from build123d import *

# Parameters (mm, degrees)
SKETCH_1_W          = 4
SKETCH_1_H          = 15
SKETCH_2_R          = 12
EXTRUDE_1_DEPTH     = 25
SKETCH_3_R          = 11
EXTRUDE_2_DEPTH     = 31
SKETCH_4_R          = 10
EXTRUDE_3_DEPTH     = 25
CUT_EXTRUDE_1_DEPTH = 3
CHAMFER_1_SIZE      = 1
FILLET_1_R          = 1


with BuildPart() as part:
    # Эскиз1 → Повернуть1 (revolve)
    with BuildSketch(Plane.XY, mode=Mode.PRIVATE) as revolve_1_sk:
        with Locations((2, 7.5)):
            Rectangle(SKETCH_1_W, SKETCH_1_H)
    revolve(revolve_1_sk.sketch.rotate(Axis((0, 0, 0), (1, 0, 0)), 270), axis=Axis((0, 0, 0), (1, 0, 0)))

    # Эскиз2 → Бобышка-Вытянуть1 (add)
    with BuildSketch(Plane(origin=(4, 0, 0), x_dir=(0, 0, -1), z_dir=(1, 0, 0))):
        Circle(SKETCH_2_R)
    extrude(amount=EXTRUDE_1_DEPTH)

    # Эскиз3 → Бобышка-Вытянуть2 (add)
    with BuildSketch(Plane(origin=(29, 0, 0), x_dir=(0, 0, -1), z_dir=(1, 0, 0))):
        Circle(SKETCH_3_R)
    extrude(amount=EXTRUDE_2_DEPTH)

    # Эскиз4 → Бобышка-Вытянуть3 (add)
    with BuildSketch(Plane(origin=(60, 0, 0), x_dir=(0, 0, -1), z_dir=(1, 0, 0))):
        Circle(SKETCH_4_R)
    extrude(amount=EXTRUDE_3_DEPTH)

    # Эскиз5 → Вырез-Вытянуть1 (cut)
    with BuildSketch(Plane(origin=(80, 0, 0), x_dir=(0, -1, 0), z_dir=(-1, 0, 0))):
        with BuildLine():
            Line((7.141428429, -7), (-7.141428429, -7))
            ThreePointArc((-7.141428429, -7), (0, -10), (7.141428429, -7))
        make_face()
    extrude(amount=-CUT_EXTRUDE_1_DEPTH, mode=Mode.SUBTRACT)

    # Фаска1
    chamfer_1_edges = [part.edges().sort_by_distance(p)[0] for p in [
        (85, 0, 10),
        (0, 0, 15),
    ]]
    chamfer(chamfer_1_edges, length=CHAMFER_1_SIZE)

    # Скругление1
    fillet_1_edges = [part.edges().sort_by_distance(p)[0] for p in [
        (4, 0, 12),
    ]]
    fillet(fillet_1_edges, radius=FILLET_1_R)


solid = part.part
For this review, take the finished solid that the model builds, in its own axes (mm). A direction names the side the tool comes from. Round coordinates to 2 decimals unless told otherwise and drop trailing zeros. Write each loop counter-clockwise with the first axis right and the second up, starting at its lowest first coordinate (ties: lowest second). Pieces come first, ordered by that corner, then holes. Notation, with made-up numbers: M 41,-31 L 69,-31 A14 cw 69,-5 Z; hole C 70.5,29.5 d3. An arc over 180 degrees is marked long. Write item = value, one per line. Start each with the question number.
(1) The part is to be moulded in two halves that separate along X. For faces 1 (the face through (80, 0, -8)), 2 (the face through (60, -10, -2)), 3 (the face through (44.28, -10.74, 2.38)), say which applies: +X half, -X half, draft (parallel to the pull), parting line (faces both ways), or undercut.
(2) We need section C-C (x = 35.5). Give the boundary of the cut face in (y, z), then the cut area to 3 significant figures.
(3) For faces 4 (the face through (2.521, 0.66, 14.985)), 5 (the face through (29, -10, -5)), 6 (the face through (81, 0, -7)), list the 3-axis set-ups (+Z, -Z, +X, -X, +Y, -Y) from which the entire face can be reached by the end or side of a thin tool; tool diameter is ignored.
(4) We need section A-A (z = 0). Give the boundary of the cut face in (x, y).
(5) For line 1 along X through (y, z) = (7, -8.25); line 2 along X through (y, z) = (6.5, -9); line 3 along Z through (x, y) = (16.5, -0.25), list the stretches that pass through material, from the lowest coordinate up.
(6) Clearance check with flat-ended pins moving along their axes: pin 1 Ø5 at (x, z) = (31.5, 8) entering from +Y; pin 2 Ø1.5 at (y, z) = (7, -11) entering from +X; pin 3 Ø10 at (x, z) = (64.5, 2.5) entering from -Y. State where each tip first meets the part, or that it passes through.
(7) We need section D-D (x = 74). Give the boundary of the cut face in (y, z).
(8) We need section B-B (y = 0). Give the boundary of the cut face in (x, z).
Results found:
q1.face_1 = undercut
q1.face_2 = +X half
q1.face_3 = draft
q2.outline = C 0,0 d22
q2.area = 380 mm²
q3.face_4 = +X, -X
q3.face_5 = +X
q3.face_6 = -Z, +Y, -Y
q4.outline = M 0,-14 L 1,-15 L 4,-15 L 4,-13 A1 cw 5,-12 L 29,-12 L 29,-11 L 60,-11 L 60,-10 L 84,-10 L 85,-9 L 85,9 L 84,10 L 60,10 L 60,11 L 29,11 L 29,12 L 5,12 A1 cw 4,13 L 4,15 L 1,15 L 0,14 Z
q5.line_1 = 0 to 60
q5.line_2 = 0 to 29
q5.line_3 = -12 to 12
q6.pin_1 = 9.53
q6.pin_2 = 4.3
q6.pin_3 = -11
q7.outline = C 0,0 d20
q8.outline = M 0,-14 L 1,-15 L 4,-15 L 4,-13 A1 cw 5,-12 L 29,-12 L 29,-11 L 60,-11 L 60,-10 L 80,-10 L 80,-7 L 83,-7 L 83,-10 L 84,-10 L 85,-9 L 85,9 L 84,10 L 60,10 L 60,11 L 29,11 L 29,12 L 5,12 A1 cw 4,13 L 4,15 L 1,15 L 0,14 Z
